Input: dimensioned drawing with shaded views. Units: mm. Origin: part minimum x, y, z. Round coordinates to 2 decimals unless told otherwise and drop trailing zeros. Loops run counter-clockwise (first coordinate to the right, second up) from the corner with the lowest first, then second, coordinate; pieces in that order, holes last. Notation, with made-up numbers: M 56.25,64 L 109.25,64 A25 ccw 109.25,85 Z; hole C 34.25,15.5 d3. An arc over 180 degrees is marked long. Answer as a JSON object with one key per item and string values.
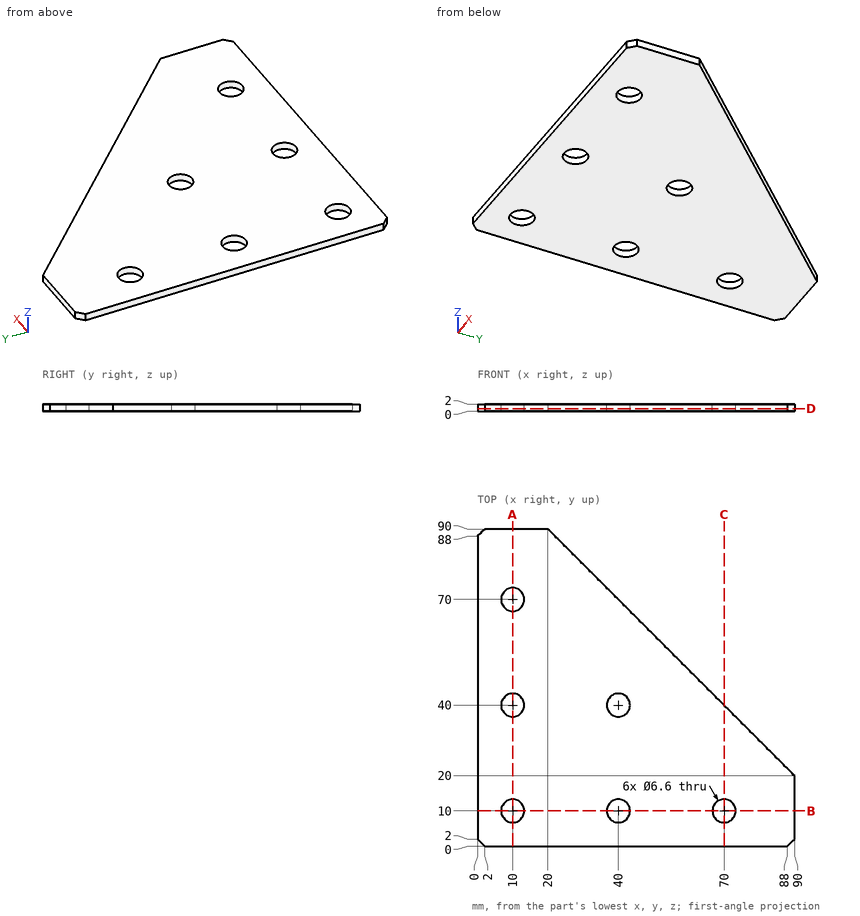
Item 1: Line query: probe 1 along X at (y, z) = (10, 1.3); probe 2 along X at (y, z) = (40, 0.65). Output: solid intervals per line, ascending. Write a range as from..to.
Answer sheet:
{"probe 1": "x = 0..6.7, 13.3..36.7, 43.3..66.7, 73.3..90", "probe 2": "x = 0..6.7, 13.3..36.7, 43.3..70"}
Item 2: Section D-D on z = 0.7. Return the cut outline in (x, y), then the cut area to 3 significant figures.
Answer sheet:
{"outline": "M 0,2 L 2,0 L 88,0 L 90,2 L 90,20 L 20,90 L 2,90 L 0,88 Z; hole C 10,10 d6.6; hole C 10,40 d6.6; hole C 10,70 d6.6; hole C 40,10 d6.6; hole C 40,40 d6.6; hole C 70,10 d6.6", "area": "5,440 mm²"}
Item 3: Section C-C on x = 70. Return the cut outline in (y, z).
Answer sheet:
{"outline": "M 0,0 L 6.7,0 L 6.7,2 L 0,2 Z; M 13.3,0 L 40,0 L 40,2 L 13.3,2 Z"}
Item 4: Section A-A on x = 10. Return the cut outline in (y, z).
Answer sheet:
{"outline": "M 0,0 L 6.7,0 L 6.7,2 L 0,2 Z; M 13.3,0 L 36.7,0 L 36.7,2 L 13.3,2 Z; M 43.3,0 L 66.7,0 L 66.7,2 L 43.3,2 Z; M 73.3,0 L 90,0 L 90,2 L 73.3,2 Z"}
